Geometry: final body of the model. Coordinates: model frame, mm. A direction names the side the tool comes from. Coordinates: 2 decimals unless noted, no trailing zeros. Write each loop counter-clockwise with the first axis right and the second up, starting at its lowest first coordinate (ties: lowest second). Pieces come first, ordered by that corner, then holes. Notation, with made-up numbers: (84, -29.5) -> (138, -29.5) arc R28 ccw to (138, -4.5) -> close; hole circle Ø3 at (13.25, 64.25). An arc over 180 degrees is marked (long way). Answer as a JSON object with one key per item and string values. Group by question number.
```python
from build123d import *

# Parameters (mm, degrees)
SKETCH_1_R      = 2.05
SKETCH_1_W      = 8.1
SKETCH_1_H      = 2.1
EXTRUDE_1_DEPTH = 2


with BuildPart() as part:
    # 草图1 → 凸台-拉伸1 (new body)
    with BuildSketch(Plane.XY):
        Polygon((-21.91868524, -9.787808432), (-21.91868524, -41.714516484), (22.419428501, -41.714516484), (22.419428501, -9.787808432), (22.419428501, 12.188083696), (-21.91868524, 53.968649146), align=None)
        with Locations((0, -35.4)):
            Circle(SKETCH_1_R, mode=Mode.SUBTRACT)
        with Locations((0, -15.4)):
            Circle(SKETCH_1_R, mode=Mode.SUBTRACT)
        with Locations((-15, -15.4)):
            Rectangle(SKETCH_1_W, SKETCH_1_H, mode=Mode.SUBTRACT)
        with Locations((15, -15.4)):
            Rectangle(SKETCH_1_W, SKETCH_1_H, mode=Mode.SUBTRACT)
    extrude(amount=EXTRUDE_1_DEPTH)


solid = part.part
```
Item 1: Ray query, L1, parallel to Y at x = 0, z = 1.25; L2, parallel to Y at x = 1.5, z = 1.8; L3, parallel to Y at x = -15, z = 0.7. Return the intervals inside material, ascending. Write a range as [from, to].
Item 2: Set-up query: faces 4 (the flat face through (-15, -14.35, 1)), 5 (the flat face through (0, -4, 2)). Return all of +Z, -Z, +X, -X, +Y, -Y with unobstructed straight access to the full face (end or side cutting, diameter ignored); none if empty.
Item 3: Section C-C on z = 1.4. Output: boundary loops of the cut face in (x, y).
Item 4: Section A-A on y = -35.4. Output: boundary loops of the cut face in (x, z).
Item 5: Contact query for flat-ended pins moving along their axis: pin 1 (1 mm diameter, centred on x = 5, z = 0.5, fed in from +Y); pin 2 (0.6 mm diameter, centred on x = 13.5, z = 1, fed in from +Y). Output: stop coordinate, or through.
Item 6: Section B-B on y = -15.4. Output: boundary loops of the cut face in (x, z), then the cut area to 3 significant figures.
Item 7: Mould query, pull axis Y, two halves, no side actions, for faces 1 (the flat face through (0, -41.715, 1)), 2 (the flat face through (-21.919, 7, 1)), 3 (the flat face through (10.95, -15, 1)). Classes: +Y half, -Y half, draft (parallel to the pull), parting line (faces both ways), or undercut.
Item 8: Section D-D on x = 0. Output: boundary loops of the cut face in (y, z), then the cut area to 3 significant figures.
Answer sheet:
{
 "1": {"L1": "y = [-41.71, -37.45], [-33.35, -17.45], [-13.35, 33.31]", "L2": "y = [-41.71, -36.8], [-34, -16.8], [-14, 31.9]", "L3": "y = [-41.71, -16.45], [-14.35, 47.45]"},
 "2": {"face 4": "+Z, -Z", "face 5": "+Z, +X, -X, +Y, -Y"},
 "3": {"outline": "(-21.92, -41.71) -> (22.42, -41.71) -> (22.42, 12.19) -> (-21.92, 53.97) -> close; hole (-19.05, -16.45) -> (-10.95, -16.45) -> (-10.95, -14.35) -> (-19.05, -14.35) -> close; hole circle Ø4.1 at (0, -35.4); hole circle Ø4.1 at (0, -15.4); hole (10.95, -16.45) -> (19.05, -16.45) -> (19.05, -14.35) -> (10.95, -14.35) -> close"},
 "4": {"outline": "(-21.92, 0) -> (-2.05, 0) -> (-2.05, 2) -> (-21.92, 2) -> close; (2.05, 0) -> (22.42, 0) -> (22.42, 2) -> (2.05, 2) -> close"},
 "5": {"pin 1": "stops at y = 29.07", "pin 2": "stops at y = 20.88"},
 "6": {"outline": "(-21.92, 0) -> (-19.05, 0) -> (-19.05, 2) -> (-21.92, 2) -> close; (-10.95, 0) -> (-2.05, 0) -> (-2.05, 2) -> (-10.95, 2) -> close; (2.05, 0) -> (10.95, 0) -> (10.95, 2) -> (2.05, 2) -> close; (19.05, 0) -> (22.42, 0) -> (22.42, 2) -> (19.05, 2) -> close", "area": "48.1 mm^2"},
 "7": {"face 1": "-Y half", "face 2": "draft", "face 3": "undercut"},
 "8": {"outline": "(-41.71, 0) -> (-37.45, 0) -> (-37.45, 2) -> (-41.71, 2) -> close; (-33.35, 0) -> (-17.45, 0) -> (-17.45, 2) -> (-33.35, 2) -> close; (-13.35, 0) -> (33.31, 0) -> (33.31, 2) -> (-13.35, 2) -> close", "area": "134 mm^2"}
}
